Geometry check sheet. Reference: drawing and pictorial views, mm from the part's lowest x, y, z. Give positions to 0.01 mm unless a question says otherwise; leave off trailing zeros. Write each loop counter-clockwise with the first axis right and the second up, starting at its lowest first coordinate (ties: lowest second). Pieces come first, ordered by that corner, then holes. Notation, with made-up numbers: (25, 15.25) -> (33, 15.25) arc R32 cw to (33, 53.25) -> close; hole circle Ø7 at (46.25, -8). An arc over 180 degrees is marked (long way). Use a Markdown table: item, result. Add a question column.
1. Scan lines: probe 1 along Y at (x, z) = (12.7, 45.5); probe 2 along Y at (x, z) = (12.7, 12.25); probe 3 along Z at (x, y) = (9, 18.75). Record each from-to range of solid material in increasing order. Write a range as [from, to].
2. Cross-section at A-A (y = 12.7). Enter the section's corners in (x, z), then the cut area to 3 significant figures.
3. Cross-section at D-D (x = 16.5). Enter the section's corners in (y, z), then the cut area to 3 significant figures.
4. Gauge pin test, flat ends, axial feed: P1, Ø12, axis at x = 21.5, z = 12, coming from the -Y side; P2, Ø1.5, axis at x = 10, z = 31.5, coming from the +Y side; P3, Ø3, axis at x = 16.5, z = 17, coming from the -Y side. Record the tip position at first contact, or that the pin passes through.
5. Cross-section at C-C (y = 16.75). Enter the section's corners in (x, z), then the cut area to 3 significant figures.
6. Release check for a two-part mould opening along Y. For the marked faces 1, 2 and 3 record: released by +Y, released by -Y, zero draft, split by the parting line, or undercut.
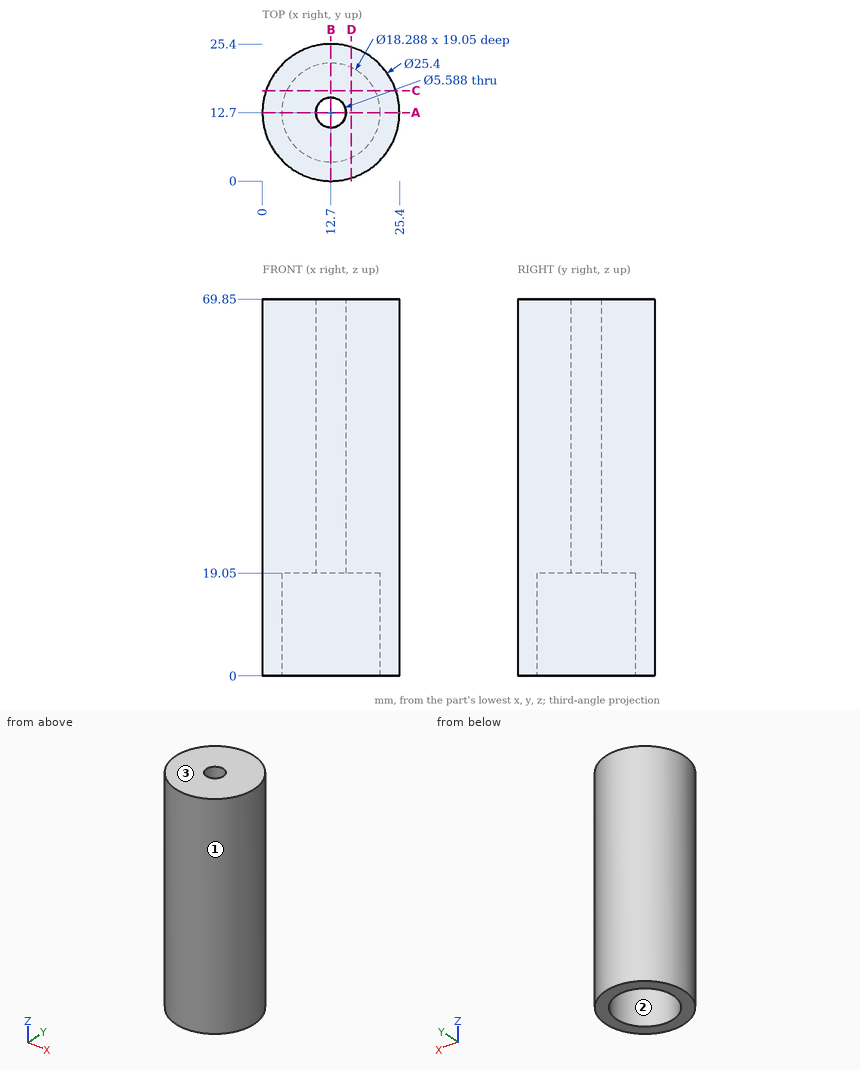
Worked answers:
| question | item | result |
|---|---|---|
| 1 | probe 1 | y = [0, 9.91], [15.49, 25.4] |
| 1 | probe 2 | y = [0, 3.56], [21.84, 25.4] |
| 1 | probe 3 | z = [19.05, 69.85] |
| 2 | outline | (0, 0) -> (3.56, 0) -> (3.56, 19.05) -> (9.91, 19.05) -> (9.91, 69.85) -> (0, 69.85) -> close; (15.49, 19.05) -> (21.84, 19.05) -> (21.84, 0) -> (25.4, 0) -> (25.4, 69.85) -> (15.49, 69.85) -> close |
| 2 | area | 1,140 mm² |
| 3 | outline | (0.58, 0) -> (4.38, 0) -> (4.38, 19.05) -> (21.02, 19.05) -> (21.02, 0) -> (24.82, 0) -> (24.82, 69.85) -> (0.58, 69.85) -> close |
| 3 | area | 1,380 mm² |
| 4 | P1 | stops at y = 0.31 |
| 4 | P2 | stops at y = 25.25 |
| 4 | P3 | stops at y = 0.21 |
| 5 | outline | (0.66, 0) -> (4.5, 0) -> (4.5, 19.05) -> (20.9, 19.05) -> (20.9, 0) -> (24.74, 0) -> (24.74, 69.85) -> (0.66, 69.85) -> close |
| 5 | area | 1,370 mm² |
| 6 | face 1 | split by the parting line |
| 6 | face 2 | undercut |
| 6 | face 3 | zero draft |
